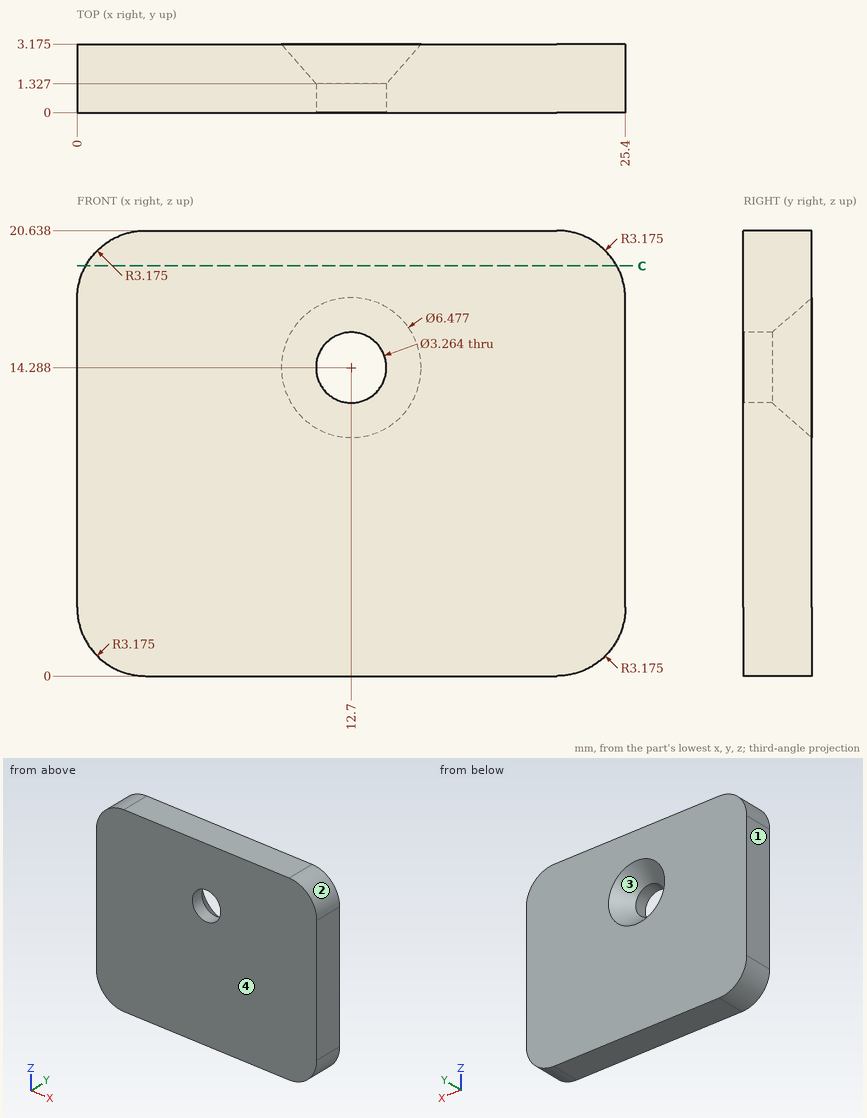
Check sheet for the drawn part. Datum: minimum x, y, z corner. Units: mm. Round coordinates to 2 decimals unless told otherwise and drop trailing zeros. Loops run counter-clockwise (first coordinate to the right, second up) from the corner with the lowest first, then second, coordinate; pieces in that order, holes last.
Item 1: Mould release check, pull along X, two halves, no side actions. Record for the marked faces 1, 2, 3 and 4: pulls with the +X half, pulls with the -X half, needs draft (parallel to the pull), parting line crosses it, or undercut.
Item 2: Thickness scan on line 1 (Z direction, x = 12.7, y = 0.8) (1 decimal); line 2 (Z direction, x = 12, y = 1.75) (1 decimal); line 3 (X direction, y = 2.85, z = 16.5). Record the ranges inside material, lowest first.
Item 3: Cross-section at C-C on z = 19. Record the boundary of the cut face in (x, y) (1 decimal).
Item 4: Gauge pin test, flat ends, axial feed: pin 1 (4 mm diameter, centred on x = 12.7, z = 14.29, fed in from +Y) (1 decimal); pin 2 (1.5 mm diameter, centred on x = 16.5, z = 13, fed in from -Y). Record the tip position at first contact, or that the pin passes through.
Answer sheet:
1. face 1: pulls with the -X half
1. face 2: pulls with the +X half
1. face 3: undercut
1. face 4: needs draft
2. line 1: z = 0 to 12.7, 15.9 to 20.6
2. line 2: z = 0 to 12.4, 16.2 to 20.6
2. line 3: x = 0 to 10.74, 14.66 to 25.4
3. outline: (0.4, 0) - (25, 0) - (25, 3.2) - (0.4, 3.2) - close
4. pin 1: stops at y = 1.8
4. pin 2: stops at y = 0
